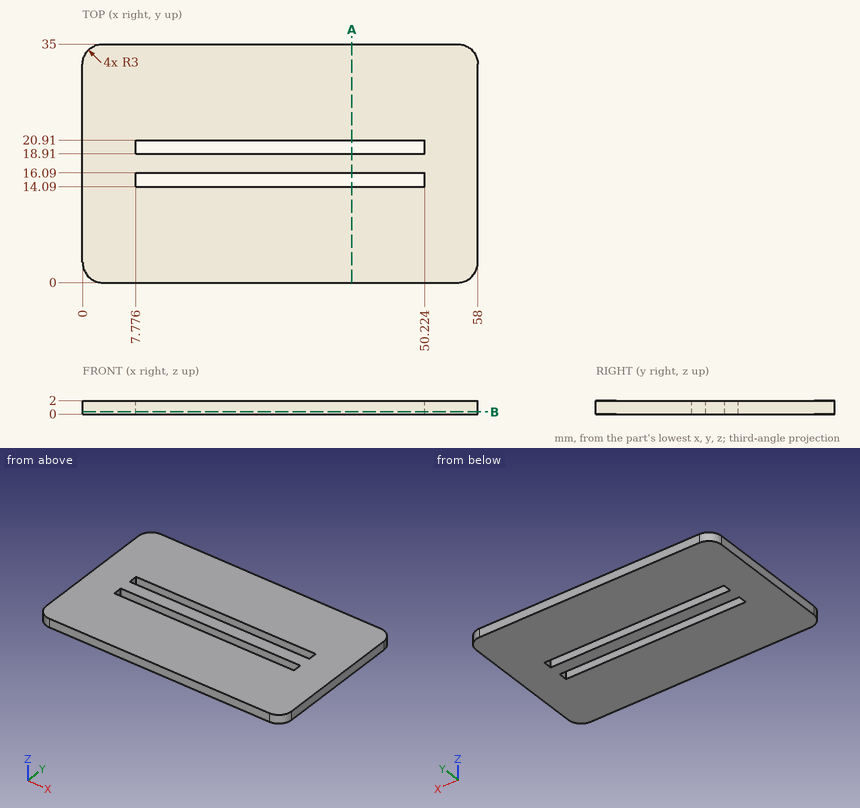
Print and shaded views of the part. All mm, measured from the part's lowest x, y and z. Coordinates: 2 decimals unless noted, no trailing zeros. Order: outer loops, then holes, each group sorted by start corner. A loop starts at its lowest first (then second) coordinate and runs counter-clockwise, first axis right, second up. Notation, with made-up numbers: (18.25, 37.5) - (47.25, 37.5) arc R14 ccw to (47.25, 59.5) - close; hole circle Ø9 at (-13, 66.5). An arc over 180 degrees is marked (long way). Return JSON: item names as keys, results as strings. Group by question number.
Item 1: Cut at B-B (z = 0.35). List the corners of the cut face in (x, y).
Item 2: Drill centre lines: probe 1 along Y at (x, z) = (31, 0.9); probe 2 along X at (y, z) = (19, 0.9); probe 3 along X at (y, z) = (1.5, 1.8). Where is each one in solid material? Low to high. Write a range as from..to.
Item 3: Cut at A-A (x = 39.5). List the corners of the cut face in (y, z), plus the area to 3 significant figures.
Check values:
{
 "1": {"outline": "(0, 3) arc R3 ccw to (3, 0) - (55, 0) arc R3 ccw to (58, 3) - (58, 32) arc R3 ccw to (55, 35) - (3, 35) arc R3 ccw to (0, 32) - close; hole (7.78, 14.09) - (50.22, 14.09) - (50.22, 16.09) - (7.78, 16.09) - close; hole (7.78, 18.91) - (50.22, 18.91) - (50.22, 20.91) - (7.78, 20.91) - close"},
 "2": {"probe 1": "y = 0..14.09, 16.09..18.91, 20.91..35", "probe 2": "x = 0..7.78, 50.22..58", "probe 3": "x = 0.4..57.6"},
 "3": {"outline": "(0, 0) - (14.09, 0) - (14.09, 2) - (0, 2) - close; (16.09, 0) - (18.91, 0) - (18.91, 2) - (16.09, 2) - close; (20.91, 0) - (35, 0) - (35, 2) - (20.91, 2) - close", "area": "62.0 mm2"}
}
